```python
from build123d import *

# Parameters (mm, degrees)
EXTRUDE_THIN1_DEPTH = 1174.75
FILLET1_R           = 1.27


with BuildPart() as part:
    # Sketch1 → Extrude-Thin1 (new body)
    with BuildSketch(Plane.XY):
        with BuildLine():
            Line((0, 0), (-4.7625, 0))
            Line((-4.7625, 0), (-4.7625, 76.2))
            Line((-4.7625, 76.2), (-7.9375, 76.2))
            Line((-7.9375, 76.2), (-7.9375, 83.154916814))
            ThreePointArc((-7.9375, 83.154916814), (-11.927152643, 94.820611714), (-22.225, 101.6))
            Line((-22.225, 101.6), (-22.225, 117.475))
            Line((-22.225, 117.475), (0, 117.475))
            Line((0, 117.475), (0, 116.205))
            Line((0, 116.205), (-20.955, 116.205))
            Line((-20.955, 116.205), (-20.955, 102.558817034))
            ThreePointArc((-20.955, 102.558817034), (-10.624694617, 95.203194699), (-6.6675, 83.154916814))
            Line((-6.6675, 83.154916814), (-6.6675, 77.47))
            Line((-6.6675, 77.47), (-3.4925, 77.47))
            Line((-3.4925, 77.47), (-3.4925, 1.27))
            Line((-3.4925, 1.27), (0, 1.27))
            Line((0, 1.27), (0, 0))
        make_face()
    extrude(amount=-EXTRUDE_THIN1_DEPTH)

    # Fillet1
    fillet1_edges = [part.edges().sort_by_distance(p)[0] for p in [
        (-3.4925, 77.47, -587.375),
        (-4.7625, 0, -587.375),
        (-7.9375, 76.2, -587.375),
        (-22.225, 101.6, -587.375),
        (-22.225, 117.475, -587.375),
    ]]
    fillet(fillet1_edges, radius=FILLET1_R)


solid = part.part
```
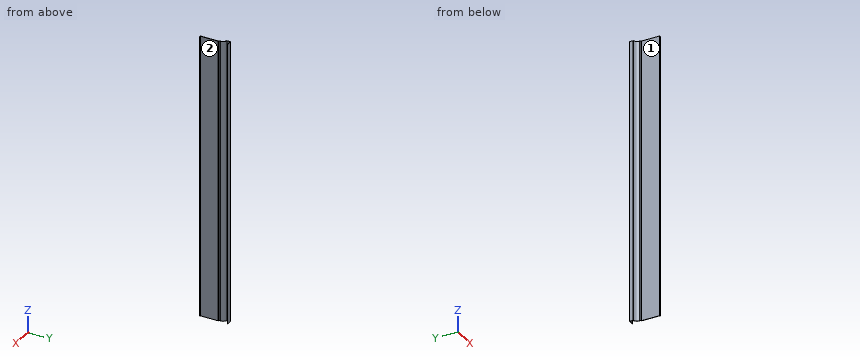
Can you work these out from the model? Positions are in its coordinate system, mm. Face numbers are marked on the shaded views. Coordinates: 2 decimals unless noted, no trailing zeros. Loops run counter-clockwise (first coordinate to the right, second up) from the corner with the lowest first, then second, coordinate; pieces in that order, holes last.
1) I need wall thicknesses on probe 1 along Y at (x, z) = (-1.75, -297) (3 decimals); probe 2 along X at (y, z) = (67, -127.5); probe 3 along Y at (x, z) = (-17, -876.5) (3 decimals). Which ranges of each line are inside material? Lowest first, please.
2) For pin 1 (1.7 mm diameter, centred on y = 79.5, z = -651, fed in from +X); pin 2 (6.5 mm diameter, centred on y = 80, z = -602.5, fed in from -X); pin 3 (3 mm diameter, centred on x = -6, z = -1035.5, fed in from -Y), each with a flat end and sliding along its axis, tell me the tip position at first contact or that it passes through.
3) Imagine slicing it at C-C on y = 47.5. List the corners of the cut face in (x, z) for me, plus the area to 3 significant figures.
4) Thinking about a two-plate mould opening in Y: for the marked faces 1 and 2, which applies, pulls with the +Y half, pulls with the -Y half, needs draft (parallel to the pull), parting line crosses it, or undercut?
Completed:
1. probe 1: y = 0 to 1.27, 116.205 to 117.475
1. probe 2: x = -4.76 to -3.49
1. probe 3: y = 99.377 to 100.851, 116.205 to 117.475
2. pin 1: stops at x = -6.67
2. pin 2: stops at x = -7.94
2. pin 3: stops at y = 0.5
3. outline: (-4.76, -1174.75) - (-3.49, -1174.75) - (-3.49, 0) - (-4.76, 0) - close
3. area: 1,490 mm2
4. face 1: needs draft
4. face 2: undercut
